For this review, use the dimensioned drawing (mm, ordinates from the lowest corner) and the shaded views. Give positions to 0.01 mm unless a question says otherwise; leave off trailing zeros. Loops run counter-clockwise (first coordinate to the right, second up) from the corner with the lowest first, then second, coordinate; pieces in that order, holes last. Notation, with made-up numbers: M 2,22.5 L 47,22.5 A20 cw 47,39.5 Z; hole C 76.25,5 d10. An arc over 180 degrees is marked long. Use one line per item in the form item = value. Start each with the question number.
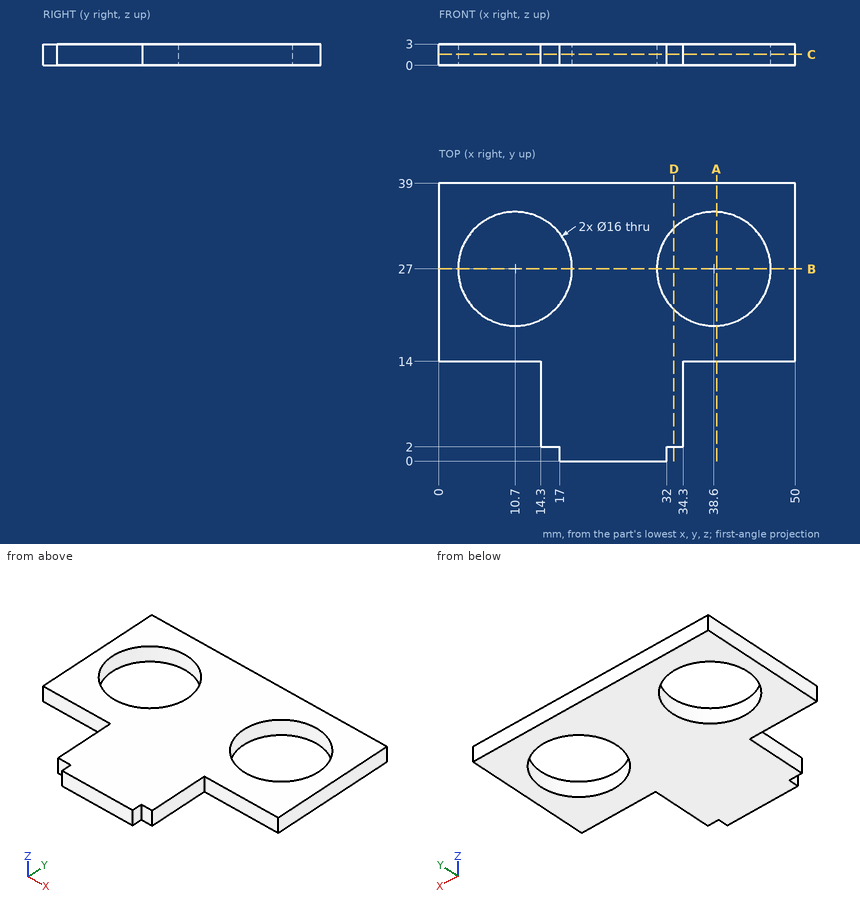
Q1. Take a section at D-D on x = 33. Give the boundary of the cut face in (y, z), plus the area to 3 significant figures.
Q2. Take a section at A-A on x = 39. Give the boundary of the cut face in (y, z).
Q3. Take a section at B-B on y = 27. Give the boundary of the cut face in (x, z), plus the area to 3 significant figures.
Q4. Wall thickness on probe 1 along X at (y, z) = (33.5, 0.8); probe 2 along Y at (x, z) = (11, 0.35); probe 3 along Y at (x, z) = (6.5, 0.25): over which ranges is each line inside the solid? List them lowest first.
Q5. Clearance check with flat-ended pins moving along their axes: pin 1 Ø1 at (y, z) = (0.5, 2) entering from -X; pin 2 Ø0.9 at (x, z) = (45.5, 1.5) entering from -Y; pin 3 Ø13 at (x, y) = (38.6, 27) entering from +Z; pin 4 Ø1.6 at (y, z) = (1, 2) entering from +X. State where each tip first meets the part, or that it passes through.
Q6. Take a section at C-C on z = 1.55. Give the boundary of the cut face in (x, y), plus the area to 3 significant figures.
Response values:
q1.outline = M 2,0 L 21.29,0 L 21.29,3 L 2,3 Z; M 32.71,0 L 39,0 L 39,3 L 32.71,3 Z
q1.area = 76.7 mm^2
q2.outline = M 14,0 L 19.01,0 L 19.01,3 L 14,3 Z; M 34.99,0 L 39,0 L 39,3 L 34.99,3 Z
q3.outline = M 0,0 L 2.7,0 L 2.7,3 L 0,3 Z; M 18.7,0 L 30.6,0 L 30.6,3 L 18.7,3 Z; M 46.6,0 L 50,0 L 50,3 L 46.6,3 Z
q3.area = 54.0 mm^2
q4.probe_1 = 0 to 6.04, 15.36 to 33.94, 43.26 to 50
q4.probe_2 = 14 to 19.01, 34.99 to 39
q4.probe_3 = 14 to 20.19, 33.81 to 39
q5.pin_1 = 17
q5.pin_2 = 14
q5.pin_3 = through
q5.pin_4 = 32
q6.outline = M 0,14 L 14.3,14 L 14.3,2 L 17,2 L 17,0 L 32,0 L 32,2 L 34.3,2 L 34.3,14 L 50,14 L 50,39 L 0,39 Z; hole C 10.7,27 d16; hole C 38.6,27 d16
q6.area = 1,120 mm^2
